Geometry check sheet. Reference: drawing and pictorial views, mm from the part's lowest x, y, z. A direction names the side the tool comes from. Coordinates: 2 decimals unless noted, no trailing zeros. Write each loop counter-clockwise with the first axis right and the second up, starting at its lowest first coordinate (ties: lowest second). Pieces come first, ordered by that corner, then holes. Notation, with made-up numbers: (-17.5, 15) -> (-6.5, 15) arc R21 cw to (-6.5, 39) -> close; hole circle Ø5 at (48, 50). An arc over 180 degrees is marked (long way). Use a Markdown table: item, result.
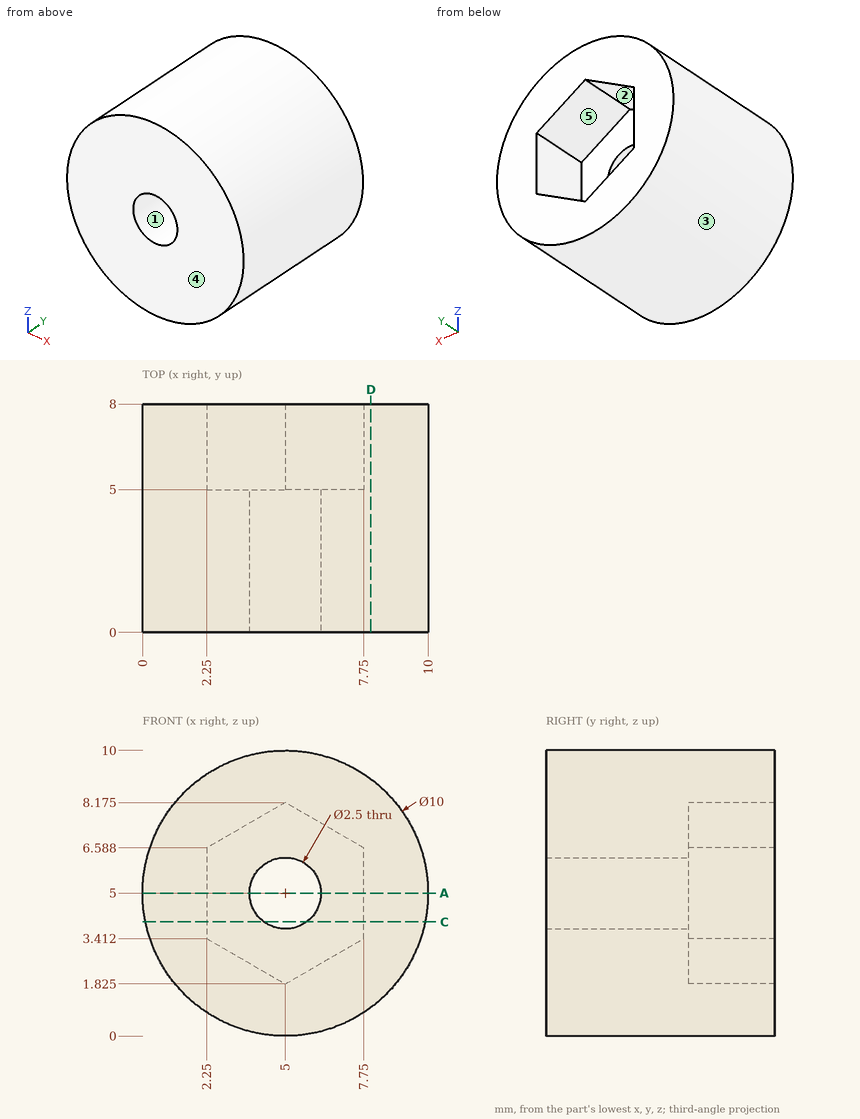
Item 1: Thickness scan on L1, parallel to Z at x = 5, y = 3.6; L2, parallel to Y at x = 4.75, z = 2.25; L3, parallel to Z at x = 7, y = 7.5. Record the ranges inside material, lowest first. Write a range as [from, to].
Answer block:
| item | result |
|---|---|
| L1 | z = [0, 3.75], [6.25, 10] |
| L2 | y = [0, 5] |
| L3 | z = [0.42, 2.98], [7.02, 9.58] |
Item 2: Section check A-A on z = 5. Record the boundary of the cut face in (x, y).
Answer block:
| item | result |
|---|---|
| outline | (0, 0) -> (3.75, 0) -> (3.75, 5) -> (2.25, 5) -> (2.25, 8) -> (0, 8) -> close; (6.25, 0) -> (10, 0) -> (10, 8) -> (7.75, 8) -> (7.75, 5) -> (6.25, 5) -> close |
Item 3: Tool access check on the marked faces 1 and 2. Record the directions out of +Z, -Z, +X, -X, +Y, -Y that give a thin tool (end or side, any length) a straight path to the whole face; none if there is none.
Answer block:
| item | result |
|---|---|
| face 1 | +Y, -Y |
| face 2 | +Y |
Item 4: Depth check by flat-ended pin: P1, Ø3, axis at y = 2, z = 2.5, coming from the +X side; P2, Ø2, axis at x = 5, z = 5, coming from the +Y side. Enter the tip coordinate at first touch or a pass-through.
Answer block:
| item | result |
|---|---|
| P1 | stops at x = 9.9 |
| P2 | passes through |
Item 5: Section check C-C on z = 4. Record the boundary of the cut face in (x, y).
Answer block:
| item | result |
|---|---|
| outline | (0.1, 0) -> (4.25, 0) -> (4.25, 5) -> (2.25, 5) -> (2.25, 8) -> (0.1, 8) -> close; (5.75, 0) -> (9.9, 0) -> (9.9, 8) -> (7.75, 8) -> (7.75, 5) -> (5.75, 5) -> close |
Item 6: Mould release check, pull along Z, two halves, no side actions. Record for the marked faces 3, 4 and 5: +Z half, -Z half, draft (parallel to the pull), parting line (faces both ways), or undercut.
Answer block:
| item | result |
|---|---|
| face 3 | parting line |
| face 4 | draft |
| face 5 | undercut |
Item 7: Section check D-D on x = 8. Record the boundary of the cut face in (y, z).
Answer block:
| item | result |
|---|---|
| outline | (0, 1) -> (8, 1) -> (8, 9) -> (0, 9) -> close |
